```python
from build123d import *

# Parameters (mm, degrees)
SKETCH1_W           = 11.6713
SKETCH1_H           = 16.51
BOSS_EXTRUDE1_DEPTH = 5.715
SKETCH2_W           = 2.385044452
SKETCH2_H           = 1.128356889
CUT_EXTRUDE1_DEPTH  = 0.254
SKETCH3_R           = 0.32385
BOSS_EXTRUDE2_DEPTH = 6.35


with BuildPart() as part:
    # Sketch1 → Boss-Extrude1 (new body)
    with BuildSketch(Plane.XY):
        Rectangle(SKETCH1_W, SKETCH1_H)
    extrude(amount=BOSS_EXTRUDE1_DEPTH)

    # Sketch2 → Cut-Extrude1 (cut)
    with BuildSketch(Plane.XY.offset(5.715)):
        with Locations((0, 7.277518213)):
            Rectangle(SKETCH2_W, SKETCH2_H)
    extrude(amount=-CUT_EXTRUDE1_DEPTH, mode=Mode.SUBTRACT)

    # Sketch3 → Boss-Extrude2 (add)
    with BuildSketch(Plane.XZ.offset(8.255)):
        with Locations((-2.6289, 2.8575)):
            Circle(SKETCH3_R)
        with Locations((0, 2.8575)):
            Circle(SKETCH3_R)
        with Locations((2.6289, 2.8575)):
            Circle(SKETCH3_R)
    extrude(amount=BOSS_EXTRUDE2_DEPTH)


solid = part.part
```
Can you work these out from the model? Positions are in its coordinate system, mm. Give positions to 0.01 mm unless a question says otherwise; leave off trailing zeros. Loops run counter-clockwise (first coordinate to the right, second up) from the corner with the lowest first, then second, coordinate; pieces in that order, holes last. Notation, with made-up numbers: M -20.75,34 L 23.25,34 A22 cw 23.25,70 Z; hole C -24,53.25 d5. An arc over 180 degrees is marked long. Use CSV: the item, a comma, the result in double quotes. Start each with the question number.
1. Imagine slicing it at D-D, the plane x = -4.25. Write out the boundary of the cut face in (y, z) (3 decimals).
2. Imagine slicing it at C-C, the plane y = -11.25. Write out the boundary of the cut face in (x, z), plus the area to 3 significant figures.
3. Imagine slicing it at A-A, the plane x = 0. Write out the boundary of the cut face in (y, z) (3 decimals).
4. If we mould it in two halves opening along Y, with no side actions, what happens to faces 1 (the face through (0, 0, 0)), 2 (the face through (0, 7, 5.461)), 3 (the face through (0, -8.255, 2)), 4 (the face through (0, 8.255, 3))? For each: released by +Y, released by -Y, zero draft, split by the parting line, or undercut.
5. Imagine slicing it at B-B, the plane z = 4.25. Write out the boundary of the cut face in (x, y) (3 decimals), plus the area to 3 significant figures.
6. If I drill on L1, parallel to Y at x = -4, z = 2 (3 decimals), over which ranges is the centre line in solid material (lowest first)?
Response values:
1,outline,"M -8.255,0 L 8.255,0 L 8.255,5.715 L -8.255,5.715 Z"
2,outline,"C -2.63,2.86 d0.65; C 0,2.86 d0.65; C 2.63,2.86 d0.65"
2,area,"0.988 mm^2"
3,outline,"M -14.605,2.534 L -8.255,2.534 L -8.255,0 L 8.255,0 L 8.255,5.715 L 7.842,5.715 L 7.842,5.461 L 6.713,5.461 L 6.713,5.715 L -8.255,5.715 L -8.255,3.181 L -14.605,3.181 Z"
4,face 1,"zero draft"
4,face 2,"undercut"
4,face 3,"released by -Y"
4,face 4,"released by +Y"
5,outline,"M -5.836,-8.255 L 5.836,-8.255 L 5.836,8.255 L -5.836,8.255 Z"
5,area,"193 mm^2"
6,L1,"-8.255 to 8.255"
